Could you check a few things on this drawing? It's one solid part, dimensions in mm from its lowest x, y, z. Round coordinates to 2 decimals unless told otherwise and drop trailing zeros. Write each loop counter-clockwise with the first axis right and the second up, starting at its lowest first coordinate (ties: lowest second). Pieces come first, ordered by that corner, then holes. Notation, with made-up numbers: (-13.75, -6.5) -> (19.25, -6.5) arc R20 ccw to (19.25, 30.5) -> close; hole circle Ø9 at (80.5, 87). An arc over 180 degrees is marked (long way). Answer as CSV lines item,"result".
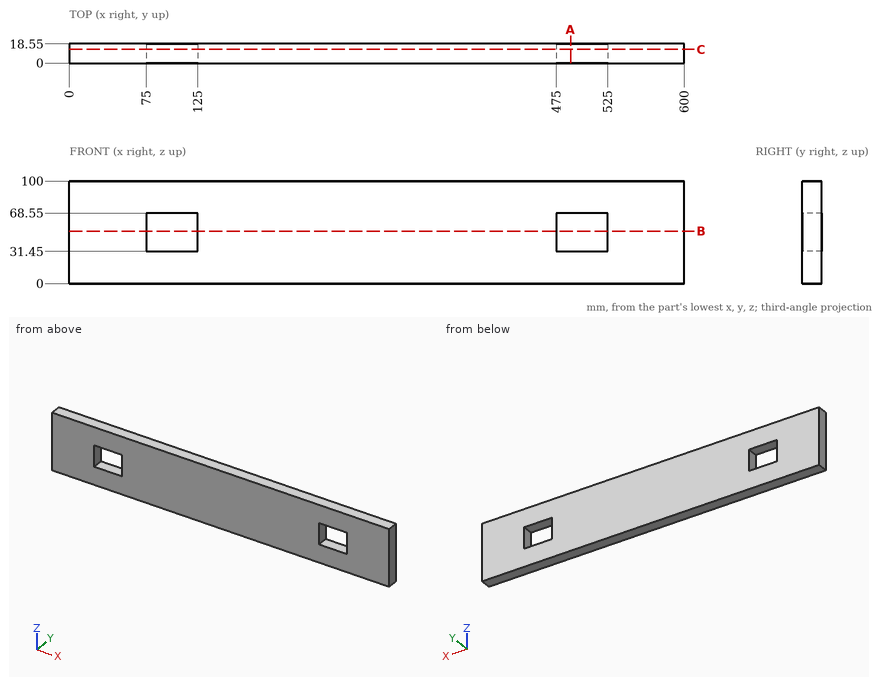
1. Suppose I cut it at B-B on z = 51. Please give me the cut outline in (x, y), and give its area (4 significant figures).
Numbers:
outline,"(0, 0) -> (75, 0) -> (75, 18.55) -> (0, 18.55) -> close; (125, 0) -> (475, 0) -> (475, 18.55) -> (125, 18.55) -> close; (525, 0) -> (600, 0) -> (600, 18.55) -> (525, 18.55) -> close"
area,"9,275 mm^2"
2. For pin 1 Ø5 at (x, y) = (227, 14) entering from -Z, with a flat end and sliding along its axis, tell me the tip position at first contact or that it passes through.
Numbers:
pin 1,"stops at z = 0"
3. Suppose I cut it at C-C on y = 13.25. Please give me the cut outline in (x, z).
Numbers:
outline,"(0, 0) -> (600, 0) -> (600, 100) -> (0, 100) -> close; hole (75, 31.45) -> (125, 31.45) -> (125, 68.55) -> (75, 68.55) -> close; hole (475, 31.45) -> (525, 31.45) -> (525, 68.55) -> (475, 68.55) -> close"
4. Suppose I cut it at A-A on x = 489. Please give me the cut outline in (y, z).
Numbers:
outline,"(0, 0) -> (18.55, 0) -> (18.55, 31.45) -> (0, 31.45) -> close; (0, 68.55) -> (18.55, 68.55) -> (18.55, 100) -> (0, 100) -> close"
5. If I drill on line 1 (X direction, y = 2.5, z = 59); line 2 (Z direction, x = 79, y = 15), over which ranges is the centre line in solid material (lowest first)?
Numbers:
line 1,"x = 0 to 75, 125 to 475, 525 to 600"
line 2,"z = 0 to 31.45, 68.55 to 100"
